Input: part model. Units: mm. Frame: model coordinates. Face numbers are marked on the shaded views. Round coordinates to 2 decimals unless told otherwise and drop trailing zeros. Order: outer loops, then holes, each group sorted by start corner. A loop starts at its lowest first (then second) coordinate and runs counter-clockwise, first axis right, second up.
Item 1: Line query: L1, parallel to X at y = -33, z = 51; L2, parallel to Y at x = -5, z = 42; L3, parallel to Z at x = 30.5, y = -29. Output: solid intervals per line, ascending.
Item 2: Mould query, pull axis X, two halves, no side actions, for the marked faces 1 and 2. Classes: released by +X, released by -X, zero draft, split by the parting line, or undercut.
Item 3: Cut plane A-A on y = -35.5. Output: boundary loops of the cut face in (x, z).
Item 4: First-contact query: pin 1 (4 mm diameter, centred on x = -42, z = 51.5, fed in from +Y); pin 2 (3 mm diameter, centred on x = 13, y = -35.5, fed in from +Z). Flat tips, straight axial feed; report the tip coordinate or a pass-through.
Item 5: Cut plane D-D on x = -35. Output: boundary loops of the cut face in (y, z).
Item 6: Cut plane C-C on y = 9. Output: boundary loops of the cut face in (x, z).
Item 7: Cut plane B-B on x = 0.5. Output: boundary loops of the cut face in (y, z), then the cut area to 3 significant figures.
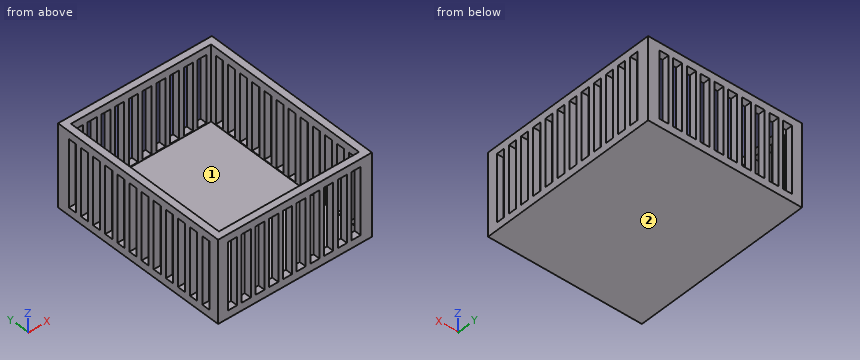
```python
from build123d import *

# Parameters (mm, degrees)
F1_W     = 111.9999963282
F1_H     = 131.9999963282
F2_DEPTH = 5
F3_W     = 111.9999963282
F3_H     = 131.9999963282
F3_W_2   = 101.9999984144
F3_H_2   = 121.9999984144
F4_DEPTH = 55
F5_W     = 3.3013222273
F5_H     = 48.7285429239
F5_W_2   = 6.6026444547
F6_DEPTH = 200
F7_W     = 2.9244981706
F7_H     = 48.8800057769
F7_W_2   = 5.8489963412
F8_DEPTH = 200


with BuildPart() as f2:
    # F1 (on face) → F2 (new body)
    with BuildSketch(Plane.XY):
        with Locations((-4.4797024012, -0.5462057889)):
            Rectangle(F1_W, F1_H)
    extrude(amount=F2_DEPTH)

    # F3 (on face) → F4 (join)
    with BuildSketch(Plane.XY.offset(5)):
        with Locations((-4.4797024012, -0.5462057889)):
            Rectangle(F3_W, F3_H)
        with Locations((-4.4797024012, -0.5462057889)):
            Rectangle(F3_W_2, F3_H_2, mode=Mode.SUBTRACT)
    extrude(amount=F4_DEPTH)

    # F5 (on face) → F6 (cut)
    with BuildSketch(Plane.XZ.offset(66.546203953)):
        with Locations((-1.6506611137, 30)):
            Rectangle(F5_W, F5_H)
        with Locations((1.6506611137, 30)):
            Rectangle(F5_W, F5_H)
        with Locations((10, 30)):
            Rectangle(F5_W_2, F5_H)
        with Locations((20, 30)):
            Rectangle(F5_W_2, F5_H)
        with Locations((30, 30)):
            Rectangle(F5_W_2, F5_H)
        with Locations((40, 30)):
            Rectangle(F5_W_2, F5_H)
        with Locations((-10, 30)):
            Rectangle(F5_W_2, F5_H)
        with Locations((-20, 30)):
            Rectangle(F5_W_2, F5_H)
        with Locations((-30, 30)):
            Rectangle(F5_W_2, F5_H)
        with Locations((-40, 30)):
            Rectangle(F5_W_2, F5_H)
        with Locations((-50, 30)):
            Rectangle(F5_W_2, F5_H)
    extrude(amount=-F6_DEPTH, mode=Mode.SUBTRACT)

    # F7 (on face) → F8 (cut)
    with BuildSketch(Plane(origin=(-60.4797005653, 0, 0), x_dir=(0, -1, 0), z_dir=(-1, 0, 0))):
        with Locations((-55.0748649985, 30)):
            Rectangle(F7_W, F7_H)
        with Locations((-52.1503668278, 30)):
            Rectangle(F7_W, F7_H)
        with Locations((-43.6126159132, 30)):
            Rectangle(F7_W_2, F7_H)
        with Locations((-33.6126159132, 30)):
            Rectangle(F7_W_2, F7_H)
        with Locations((-23.6126159132, 30)):
            Rectangle(F7_W_2, F7_H)
        with Locations((-13.6126159132, 30)):
            Rectangle(F7_W_2, F7_H)
        with Locations((-3.6126159132, 30)):
            Rectangle(F7_W_2, F7_H)
        with Locations((6.3873840868, 30)):
            Rectangle(F7_W_2, F7_H)
        with Locations((16.3873840868, 30)):
            Rectangle(F7_W_2, F7_H)
        with Locations((26.3873840868, 30)):
            Rectangle(F7_W_2, F7_H)
        with Locations((36.3873840868, 30)):
            Rectangle(F7_W_2, F7_H)
        with Locations((46.3873840868, 30)):
            Rectangle(F7_W_2, F7_H)
        with Locations((56.3873840868, 30)):
            Rectangle(F7_W_2, F7_H)
    extrude(amount=-F8_DEPTH, mode=Mode.SUBTRACT)


solid = f2.part
```
From the geometry:
1. L1: x = -60.48 to -55.48, 46.52 to 51.52
1. L2: y = -66.55 to -61.55, 60.45 to 65.45
1. L3: z = 0 to 5
2. face 1: undercut
2. face 2: zero draft
3. outline: (-60.48, 0) - (51.52, 0) - (51.52, 5.56) - (46.52, 5.56) - (46.52, 5) - (-55.48, 5) - (-55.48, 5.56) - (-60.48, 5.56) - close; (-60.48, 54.44) - (-55.48, 54.44) - (-55.48, 60) - (-60.48, 60) - close; (46.52, 54.44) - (51.52, 54.44) - (51.52, 60) - (46.52, 60) - close
4. pin 1: stops at y = 65.45
4. pin 2: stops at z = 5
5. outline: (-66.55, 0) - (65.45, 0) - (65.45, 60) - (60.45, 60) - (60.45, 5) - (-61.55, 5) - (-61.55, 60) - (-66.55, 60) - close
6. outline: (-60.48, 0) - (51.52, 0) - (51.52, 60) - (46.52, 60) - (46.52, 5) - (-55.48, 5) - (-55.48, 60) - (-60.48, 60) - close
7. outline: (-66.55, 0) - (65.45, 0) - (65.45, 5.64) - (60.45, 5.64) - (60.45, 5) - (-61.55, 5) - (-61.55, 5.64) - (-66.55, 5.64) - close; (-66.55, 54.36) - (-61.55, 54.36) - (-61.55, 60) - (-66.55, 60) - close; (60.45, 54.36) - (65.45, 54.36) - (65.45, 60) - (60.45, 60) - close
7. area: 723 mm2
